Verification items for this drawing (mm, ordinates from the low corner). Round coordinates to 2 decimals unless told otherwise and drop trailing zeros. Loops run counter-clockwise (first coordinate to the right, second up) from the corner with the lowest first, then second, coordinate; pieces in that order, holes last. Notation, with made-up numbers: M -23.5,68 L 14.5,68 A19 ccw 14.5,101 Z; hole C 0,-25.5 d8. An arc over 180 degrees is marked long. Write item = value, one per line.
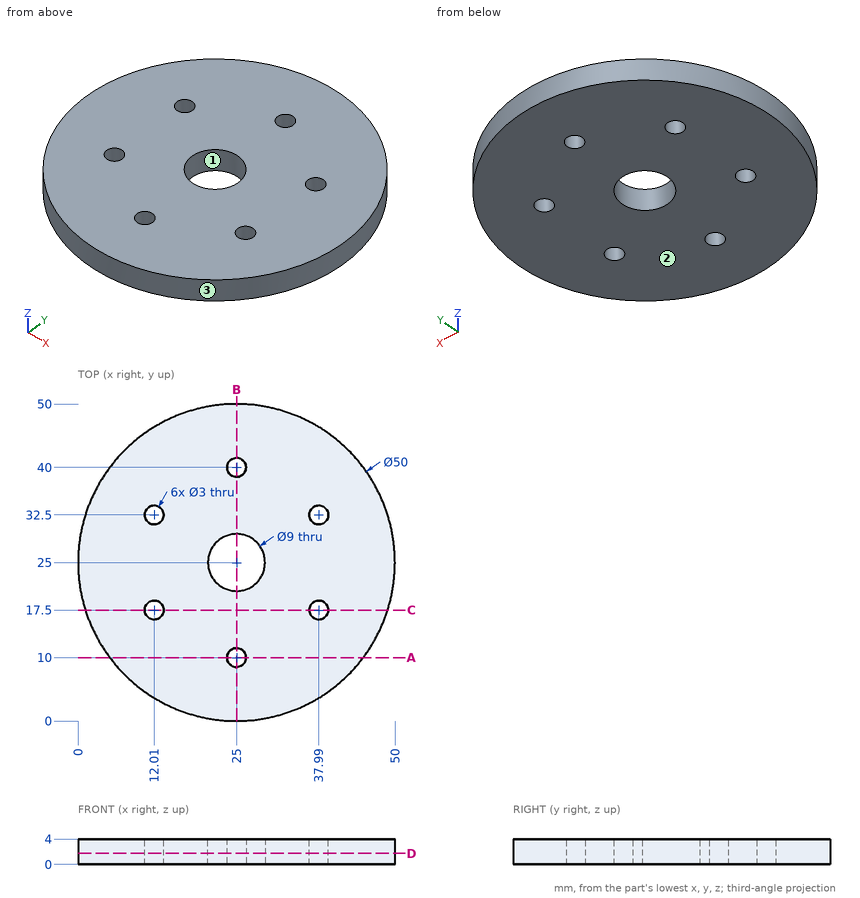
(1) Material ranges on line 1 along Y through (x, z) = (25, 1.75); line 2 along Y through (x, z) = (38, 2.75) (1 decimal); line 3 along Y through (x, z) = (26, 0.65), recorded low to high. Write a range as from..to.
Result set:
line_1 = 0..8.5, 11.5..20.5, 29.5..38.5, 41.5..50
line_2 = 3.6..16, 19..31, 34..46.4
line_3 = 0.02..8.88, 11.12..20.61, 29.39..38.88, 41.12..49.98
(2) Sectioned sample at D-D on z = 1.75. Record the cut outline in (x, y), then the cut area to 3 significant figures.
Result set:
outline = C 25,25 d50; hole C 12.01,17.5 d3; hole C 12.01,32.5 d3; hole C 25,25 d9; hole C 25,10 d3; hole C 25,40 d3; hole C 37.99,17.5 d3; hole C 37.99,32.5 d3
area = 1,860 mm2
(3) Sectioned sample at B-B on x = 25. Record the cut outline in (y, z).
Result set:
outline = M 0,0 L 8.5,0 L 8.5,4 L 0,4 Z; M 11.5,0 L 20.5,0 L 20.5,4 L 11.5,4 Z; M 29.5,0 L 38.5,0 L 38.5,4 L 29.5,4 Z; M 41.5,0 L 50,0 L 50,4 L 41.5,4 Z
(4) Sectioned sample at A-A on y = 10. Record the cut outline in (x, z).
Result set:
outline = M 5,0 L 23.5,0 L 23.5,4 L 5,4 Z; M 26.5,0 L 45,0 L 45,4 L 26.5,4 Z
(5) Sectioned sample at C-C on y = 17.5. Record the cut outline in (x, z), then the cut area to 3 significant figures.
Result set:
outline = M 1.15,0 L 10.51,0 L 10.51,4 L 1.15,4 Z; M 13.51,0 L 36.49,0 L 36.49,4 L 13.51,4 Z; M 39.49,0 L 48.85,0 L 48.85,4 L 39.49,4 Z
area = 167 mm2
(6) Release check for a two-part mould opening along Y. For the marked faces 1, 2 and 3 record: released by +Y, released by -Y, zero draft, split by the parting line, or undercut.
Result set:
face_1 = undercut
face_2 = zero draft
face_3 = split by the parting line
(7) Depth check by flat-ended pin: pin 1 Ø2 at (x, z) = (37, 1) entering from +Y; pin 2 Ø8 at (x, y) = (25, 25) entering from +Z; pin 3 Ø1 at (x, z) = (16.5, 2) entering from +Y (1 decimal); pin 4 Ø1.5 at (x, z) = (30, 2.5) entering from +Y. Enter the tip coordinate at first touch or a pass-through.
Result set:
pin_1 = 47.45
pin_2 = through
pin_3 = 48.7
pin_4 = 49.64
